Read the model definition and answer for the solid it produces. Units are mm, in the model's axes. Face numbers are marked on the shaded views. A direction names the side the tool comes from. Give positions to 0.01 mm unless a question says otherwise; leave off trailing zeros. Order: outer loops, then holes, each group sorted by start corner. A loop starts at its lowest first (then second) coordinate and runs counter-clockwise, first axis right, second up. Notation, with made-up numbers: (52.5, -20.5) -> (63.5, -20.5) arc R26 cw to (63.5, -2.5) -> close; hole circle Ø6 at (52, 4.25). An arc over 180 degrees is marked (long way). One line per question, with ' | ' between items. Start each with the question number.
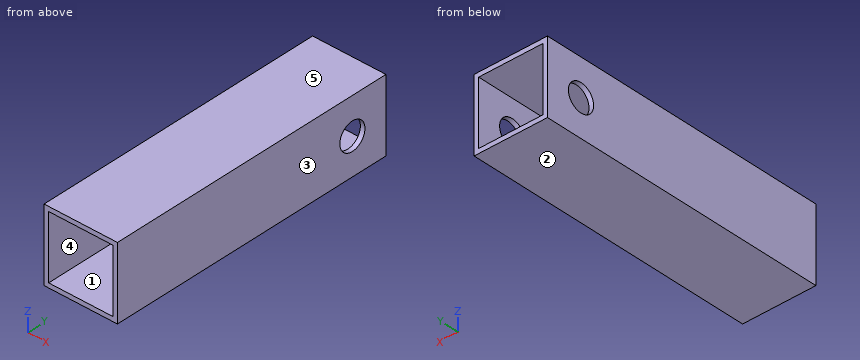
Autodesk Inventor part; units mm, degrees
ref_plane "YZ Plane" through (0, 0, 0) normal (1, 0, 0) x (0, 1, 0)
ref_plane "XZ Plane" through (0, 0, 0) normal (0, 1, 0) x (-1, 0, 0)
ref_plane "XY Plane" through (0, 0, 0) normal (0, 0, 1) x (1, 0, 0)
sketch "Sketch1" plane through (0, 0, 0) normal (0, 0, 1) x (1, 0, 0)
  line L0 (0, 0) -> (25.4, 0)
  line L1 (25.4, 0) -> (25.4, 101.6)
  line L2 (25.4, 101.6) -> (0, 101.6)
  line L3 (0, 101.6) -> (0, 0)
  dimension "d0" = 25.4
  dimension "d1" = 101.6
extrude "Extrusion1" add sketch "Sketch1" along normal blind 25.4
shell "Shell1" thickness 1.5875 removed faces 2 at (16.9333, 101.6, 16.9333) at (8.4667, 0, 8.4667)
sketch "Sketch2" plane through (25.4, 0, 0) normal (1, 0, 0) x (0, 0, -1)
  line L0 (0, 0) -> (0, 101.6)
  line L1 (0, 101.6) -> (-25.4, 101.6)
  circle A0 centre (-12.7, 88.9) radius 4.7625
  dimension "d5" = 9.525
  dimension "d6" = 12.7
  dimension "d7" = 12.7
extrude "Extrusion2" cut sketch "Sketch2" against normal through all
properties part number "VerticalRail" material "Aluminum-6061"
Q1. A cutting plane is placed at C-C, the plane y = 88.9. Determine the outline of the cut face in (x, z), then the cut area to 3 significant figures.
Q2. A cutting plane is placed at D-D, the plane z = 4.75. Determine the outline of the cut face in (x, y), then the cut area to 3 significant figures.
Q3. Which of the six approach directions +Z, -Z, +X, -X, +Y, -Y give full straight-line access (tool end or side, diameter ignored) to the marked faces 4 and 5?
Q4. A cutting plane is placed at A-A, the plane z = 12.7. Determine the outline of the cut face in (x, y).
Q5. Given P1, Ø10, axis at x = 9, z = 9.5, coming from the -Y side, flat-ended and moving along its own axis, determine where the tip first touches the part or whether it passes through.
Q6. A cutting plane is placed at B-B, the plane x = 14. Determine the outline of the cut face in (y, z).
Q7. Determine the mould class of the marked faces 1, 2 and 3 for opening direction X: pulls with the +X half, pulls with the -X half, needs draft (parallel to the pull), parting line crosses it, or undercut.
Q8. Find the intervals of material crossed by line 1 (X direction, y = 48.5, z = 13); line 2 (Y direction, x = 1, z = 12.7), in increasing order.
Geometry results:
1) outline: (0, 0) -> (25.4, 0) -> (25.4, 7.94) -> (23.81, 7.94) -> (23.81, 1.59) -> (1.59, 1.59) -> (1.59, 7.94) -> (0, 7.94) -> close; (0, 17.46) -> (1.59, 17.46) -> (1.59, 23.81) -> (23.81, 23.81) -> (23.81, 17.46) -> (25.4, 17.46) -> (25.4, 25.4) -> (0, 25.4) -> close | area: 121 mm²
2) outline: (0, 0) -> (1.59, 0) -> (1.59, 101.6) -> (0, 101.6) -> close; (23.81, 0) -> (25.4, 0) -> (25.4, 101.6) -> (23.81, 101.6) -> close | area: 323 mm²
3) face 4: +Y, -Y | face 5: +Z, +X, -X, +Y, -Y
4) outline: (0, 0) -> (1.59, 0) -> (1.59, 84.14) -> (0, 84.14) -> close; (0, 93.66) -> (1.59, 93.66) -> (1.59, 101.6) -> (0, 101.6) -> close; (23.81, 0) -> (25.4, 0) -> (25.4, 84.14) -> (23.81, 84.14) -> close; (23.81, 93.66) -> (25.4, 93.66) -> (25.4, 101.6) -> (23.81, 101.6) -> close
5) P1: through
6) outline: (0, 0) -> (101.6, 0) -> (101.6, 1.59) -> (0, 1.59) -> close; (0, 23.81) -> (101.6, 23.81) -> (101.6, 25.4) -> (0, 25.4) -> close
7) face 1: undercut | face 2: needs draft | face 3: pulls with the +X half
8) line 1: 0 to 1.59, 23.81 to 25.4 | line 2: 0 to 84.14, 93.66 to 101.6
